Geometry check sheet. Reference: the model listing, model coordinates, mm. Face numbers are marked on the shaded views. Give positions to 0.01 mm unless a question says otherwise; leave off trailing zeros. Write each loop counter-clockwise with the first axis right and the second up, starting at its lowest first coordinate (ties: lowest second). Pieces come first, ordered by that corner, then holes.
(1) Cross-section at B-B (y = -9.5). Record the boundary of the cut face in (x, z), and give its area (3 significant figures).
(2) Cross-section at A-A (z = -2). Record the boundary of the cut face in (x, y).
(3) Cross-section at D-D (y = -21). Record the boundary of the cut face in (x, z), and give its area (3 significant figures).
(4) Depth check by flat-ended pin: P1, Ø1.4, axis at x = -43, y = -1, coming from the -Z side; P2, Ø1.2, axis at y = 26.5, z = -1, coming from the +X side; P3, Ø4, axis at y = -10, z = 2.5, coming from the +X side; P4, Ø3.5, axis at x = -8.5, z = -1, coming from the -Y side. Enter the tip coordinate at first touch or a pass-through.
(5) Mould release check, pull along Z, two halves, no side actions. Record for the marked faces 1 and 2: +Z half, -Z half, draft (parallel to the pull), parting line (faces both ways), or undercut.
(6) Cross-section at C-C (x = 12). Record the boundary of the cut face in (y, z), and give its area (4 significant figures).
(7) Thickness scan on line 1 along X through (y, z) = (7, -2); line 2 along Y through (x, z) = (-42.5, 4.25); line 3 along X through (y, z) = (-2, 0.5). Record the ranges inside material, lowest first.
```python
from build123d import *
from OCP.BRepFilletAPI import BRepFilletAPI_MakeChamfer

# Parameters (mm, degrees)
SKETCH1_R           = 0.925
BOSS_EXTRUDE1_DEPTH = 5
BOSS_EXTRUDE2_DEPTH = 3
SKETCH7_W           = 9
SKETCH7_H           = 9
CUT_EXTRUDE3_DEPTH  = 47.770717335
SKETCH3_R           = 2.25
BOSS_EXTRUDE3_DEPTH = 5
SKETCH4_R           = 3.5
CUT_EXTRUDE1_DEPTH  = 3
CHAMFER2_SIZE       = 5.1
FILLET1_R           = 7
CHAMFER3_SIZE       = 0.5
CHAMFER1_SIZE       = 1.25
CHAMFER1_SIZE_2     = 2.5


with BuildPart() as part:
    # Sketch1 → Boss-Extrude1 (new body)
    with BuildSketch(Plane.XY):
        Polygon((-30, -25), (-30, 20), (30, 20), (30, -25), (37.5, -25), (37.5, 27.5), (-37.5, 27.5), (-37.5, -25), align=None)
        with Locations((-33, 23)):
            Circle(SKETCH1_R, mode=Mode.SUBTRACT)
        with Locations((33, 23)):
            Circle(SKETCH1_R, mode=Mode.SUBTRACT)
    extrude(amount=BOSS_EXTRUDE1_DEPTH)

    # Sketch2 → Boss-Extrude2 (add)
    with BuildSketch(Plane.XY):
        Polygon((37.5, 27.5), (30, 27.5), (-30, 27.5), (-37.5, 27.5), (-37.5, -25), (-35.1, -25), (-35.1, 25.1), (35.1, 25.1), (35.1, -25), (37.5, -25), align=None)
    extrude(amount=-BOSS_EXTRUDE2_DEPTH)

    # Sketch7 → Cut-Extrude3 (cut, through all)
    with BuildSketch(Plane(origin=(0, 0, 0), x_dir=(-1, 0, 0), z_dir=(0, 0, -1))):
        with Locations((-33, 23)):
            Rectangle(SKETCH7_W, SKETCH7_H)
        with Locations((33, 23)):
            Rectangle(SKETCH7_W, SKETCH7_H)
    extrude(amount=CUT_EXTRUDE3_DEPTH, mode=Mode.SUBTRACT)

    # Sketch3 → Boss-Extrude3 (add)
    # profile 1 of 2: a face of its own
    with BuildSketch(Plane.XY):
        with BuildLine():
            Line((42.5, 5), (37.5, 5))
            Line((37.5, 5), (37.5, -5))
            Line((37.5, -5), (42.5, -5))
            ThreePointArc((42.5, -5), (47.5, 0), (42.5, 5))
        make_face()
        with Locations(Location((42.5, 0, 0), (0, 0, 180))):
            Circle(SKETCH3_R, mode=Mode.SUBTRACT)
    # profile 2 of 2: a face of its own
    with BuildSketch(Plane.XY):
        with BuildLine():
            Line((-42.5, 5), (-37.5, 5))
            Line((-37.5, 5), (-37.5, -5))
            Line((-37.5, -5), (-42.5, -5))
            ThreePointArc((-42.5, -5), (-47.5, 0), (-42.5, 5))
        make_face()
        with Locations(Location((-42.5, 0, 0), (0, 0, 180))):
            Circle(SKETCH3_R, mode=Mode.SUBTRACT)
    extrude(amount=BOSS_EXTRUDE3_DEPTH)

    # Sketch4 → Cut-Extrude1 (cut)
    with BuildSketch(Plane(origin=(0, 0, 0), x_dir=(-1, 0, 0), z_dir=(0, 0, -1))):
        with Locations((-42.5, 0)):
            Circle(SKETCH4_R)
        with Locations((42.5, 0)):
            Circle(SKETCH4_R)
    extrude(amount=-CUT_EXTRUDE1_DEPTH, mode=Mode.SUBTRACT)

    # Chamfer2
    chamfer2_edges = [part.edges().sort_by_distance(p)[0] for p in [
        (-30, -25, 2.5),
        (30, -25, 2.5),
    ]]
    chamfer(chamfer2_edges, length=CHAMFER2_SIZE)

    # Fillet1
    fillet1_edges = [part.edges().sort_by_distance(p)[0] for p in [
        (-37.5, 27.5, 2.5),
        (37.5, 27.5, 2.5),
    ]]
    fillet(fillet1_edges, radius=FILLET1_R)

    # Chamfer3
    chamfer3_edges = [part.edges().sort_by_distance(p)[0] for p in [
        (37.5, 12.75, 5),
        (47.5, 0, 5),
        (40, 5, 5),
        (40, -5, 5),
        (44.75, 0, 5),
        (-37.5, -15, 5),
        (-47.5, 0, 5),
        (-40, -5, 5),
        (-40, 5, 5),
        (-40.25, 0, 5),
        (0, 20, 5),
        (-30, 0.05, 5),
        (36.3, -25, 5),
        (32.55, -22.45, 5),
        (-32.55, -22.45, 5),
        (-37.5, 12.75, 5),
        (0, 27.5, 5),
        (35.449747468, 25.449747468, 5),
        (-35.449747468, 25.449747468, 5),
        (30, 0.05, 5),
        (-33.925, 23, 0),
        (-33.925, 23, 5),
        (37.5, -15, 5),
        (32.075, 23, 0),
        (32.075, 23, 5),
        (-36.3, -25, 5),
    ]]
    chamfer(chamfer3_edges, length=CHAMFER3_SIZE)

    # Chamfer1
    chamfer1_edges_1 = [part.edges().sort_by_distance(p)[0] for p in [
        (46, 0, 3),
    ]]
    chamfer1_side_1 = [part.faces().sort_by_distance(p)[0] for p in [
        (45.975, 0, 3),
    ]]
    chamfer1_edges_2 = [part.edges().sort_by_distance(p)[0] for p in [
        (-39, 0, 3),
    ]]
    chamfer1_side_2 = [part.faces().sort_by_distance(p)[0] for p in [
        (-39.025, 0, 3),
    ]]
    chamfer1 = BRepFilletAPI_MakeChamfer(part.part.solid().wrapped)
    for e in chamfer1_edges_1:
        chamfer1.Add(CHAMFER1_SIZE - 0.0001, CHAMFER1_SIZE_2 - 0.0001, e.wrapped, chamfer1_side_1[0].wrapped)
    for e in chamfer1_edges_2:
        chamfer1.Add(CHAMFER1_SIZE - 0.0001, CHAMFER1_SIZE_2 - 0.0001, e.wrapped, chamfer1_side_2[0].wrapped)
    add(Compound.cast(chamfer1.Shape()), mode=Mode.REPLACE)  # a hair under: the kernel refuses the full size


solid = part.part
```
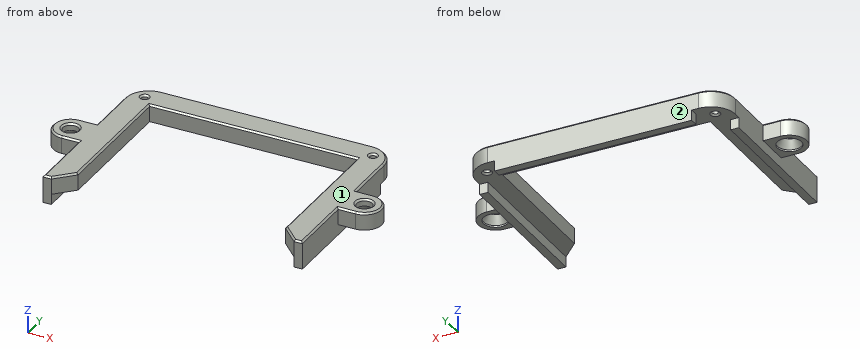
Reply:
1. outline: (-37.5, -3) - (-35.1, -3) - (-35.1, 0) - (-30, 0) - (-30, 4.5) - (-30.5, 5) - (-37, 5) - (-37.5, 4.5) - close; (30, 0) - (35.1, 0) - (35.1, -3) - (37.5, -3) - (37.5, 4.5) - (37, 5) - (30.5, 5) - (30, 4.5) - close
1. area: 88.9 mm2
2. outline: (-37.5, -25) - (-35.1, -25) - (-35.1, 18.5) - (-37.5, 18.5) - close; (-28.5, 25.1) - (28.5, 25.1) - (28.5, 27.5) - (-28.5, 27.5) - close; (35.1, -25) - (37.5, -25) - (37.5, 18.5) - (35.1, 18.5) - close
3. outline: (-37.5, -3) - (-35.1, -3) - (-35.1, 0) - (-31.1, 0) - (-31.1, 4.5) - (-31.81, 5) - (-37, 5) - (-37.5, 4.5) - close; (31.1, 0) - (35.1, 0) - (35.1, -3) - (37.5, -3) - (37.5, 4.5) - (37, 5) - (31.81, 5) - (31.1, 4.5) - close
3. area: 77.8 mm2
4. P1: passes through
4. P2: stops at x = 28.5
4. P3: stops at x = 37.5
4. P4: stops at y = 20
5. face 1: +Z half
5. face 2: draft
6. outline: (20, 0) - (25.1, 0) - (25.1, -3) - (27.5, -3) - (27.5, 4.5) - (27, 5) - (20.5, 5) - (20, 4.5) - close
6. area: 44.45 mm2
7. line 1: x = -37.5 to -35.1, 35.1 to 37.5
7. line 2: y = -5 to -2.25, 2.25 to 5
7. line 3: x = -47.08 to -45.37, -39.63 to -30, 30 to 39.63, 45.37 to 47.08
